```python
from build123d import *

# Parameters (mm, degrees)
SKETCH2_W           = 50
SKETCH2_H           = 15
BOSS_EXTRUDE1_DEPTH = 2
SKETCH4_W           = 46
SKETCH4_H           = 11
BOSS_EXTRUDE2_DEPTH = 2
SKETCH5_W           = 43.009657984
SKETCH5_H           = 9.00272897
CUT_EXTRUDE1_DEPTH  = 1


with BuildPart() as part:
    # Sketch2 → Boss-Extrude1 (new body)
    with BuildSketch(Plane(origin=(0, 0, 0), x_dir=(0, 0, -1), z_dir=(1, 0, 0))):
        with Locations((-3.923357664, -3.48540146)):
            Rectangle(SKETCH2_W, SKETCH2_H)
    extrude(amount=BOSS_EXTRUDE1_DEPTH)

    # Sketch4 → Boss-Extrude2 (add)
    with BuildSketch(Plane(origin=(2, 0, 0), x_dir=(0, 0, -1), z_dir=(1, 0, 0))):
        with Locations((-3.923357664, -3.48540146)):
            Rectangle(SKETCH4_W, SKETCH4_H)
    extrude(amount=BOSS_EXTRUDE2_DEPTH)

    # Sketch5 → Cut-Extrude1 (cut)
    with BuildSketch(Plane(origin=(4, 0, 0), x_dir=(0, 0, -1), z_dir=(1, 0, 0))):
        with Locations((-3.928186656, -3.486765945)):
            Rectangle(SKETCH5_W, SKETCH5_H)
    extrude(amount=-CUT_EXTRUDE1_DEPTH, mode=Mode.SUBTRACT)


solid = part.part
```
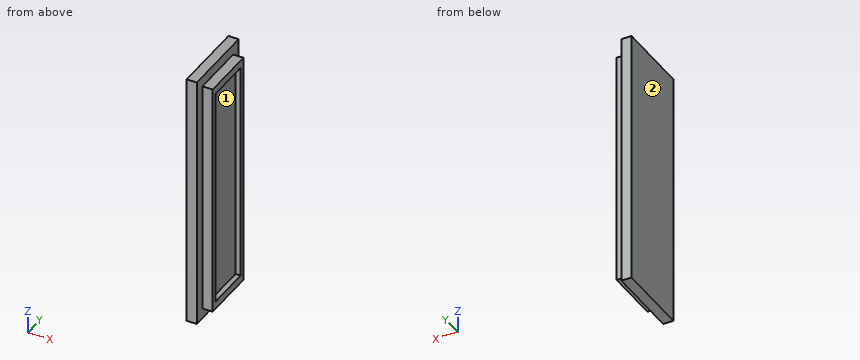
For this review, take the finished solid that the model builds, in its own axes (mm). Face numbers are marked on the shaded views. Round coordinates to 2 decimals unless told otherwise and drop trailing zeros. Loops run counter-clockwise (first coordinate to the right, second up) from the corner with the lowest first, then second, coordinate; pieces in that order, holes last.
Q1. Add section A-A on y = -8.5. Write out the cut boundary in (x, z), plus the area to 3 significant figures.
Result sheet:
outline: (0, -21.08) - (2, -21.08) - (2, -19.08) - (4, -19.08) - (4, 26.92) - (2, 26.92) - (2, 28.92) - (0, 28.92) - close
area: 192 mm2
Q2. To check wall thickness, follow line 1 along Y through (x, z) = (3.85, 12.5); line 2 along Z through (x, y) = (3.65, -2.5); line 3 along Y through (x, z) = (2.25, -13.5). State the ranges of each line that lie inside material, in increasing order.
Result sheet:
line 1: y = -8.99 to -7.99, 1.01 to 2.01
line 2: z = -19.08 to -17.58, 25.43 to 26.92
line 3: y = -8.99 to 2.01
Q3. Insertion check: pin 1 Ø0.8 at (x, z) = (3.5, 12) entering from +Y; pin 2 Ø1 at (x, y) = (3.5, -6) entering from +Z; pin 3 Ø7 at (y, z) = (-4, 7) entering from +X. Each pin has a flat end and moves straight along its axis. Give the tip position at first contact, or say it passes through.
Result sheet:
pin 1: stops at y = 2.01
pin 2: stops at z = 26.92
pin 3: stops at x = 3
Q4. Mouldability with a two-part tool opening along X and no side actions: class the marked faces 1 and 2 as +X half, -X half, draft (parallel to the pull), parting line (faces both ways), or undercut.
Result sheet:
face 1: +X half
face 2: -X half
Q5. Add section C-C on z = -6.5. Write out the cut boundary in (x, y).
Result sheet:
outline: (0, -10.99) - (2, -10.99) - (2, -8.99) - (4, -8.99) - (4, -7.99) - (3, -7.99) - (3, 1.01) - (4, 1.01) - (4, 2.01) - (2, 2.01) - (2, 4.01) - (0, 4.01) - close
Q6. Add section B-B on x = 3.5. Write out the cut boundary in (y, z).
Result sheet:
outline: (-8.99, -19.08) - (2.01, -19.08) - (2.01, 26.92) - (-8.99, 26.92) - close; hole (-7.99, -17.58) - (1.01, -17.58) - (1.01, 25.43) - (-7.99, 25.43) - close
